Design review of the part built by this model. Coordinates are the model's own, in mm. Face numbers are marked on the shaded views. A direction names the side the tool comes from. Give positions to 0.01 mm unless a question says otherwise; leave off trailing zeros. Loops run counter-clockwise (first coordinate to the right, second up) from the corner with the lowest first, then second, coordinate; pieces in that order, holes last. Notation, with made-up numbers: M 72.5,77.25 L 127.5,77.25 A22 ccw 127.5,99.25 Z; hole C 18.5,14 d6. An arc over 180 degrees is marked long. Use one line per item in the form item = value. Start each with the question number.
from build123d import *

# Parameters (mm, degrees)
F0_W     = 22
F0_H     = 10
F1_DEPTH = 10
F2_R     = 1.65
F2_W     = 7
F2_H     = 4
F3_DEPTH = 10.001
F4_R     = 4.99999


# Not quite as in the source:
# - a fillet or chamfer is up to 0.001 mm smaller than in the source, because OpenCascade refuses the exact size


with BuildPart() as f1:
    # F0 (on Top) → F1 (new body)
    with BuildSketch(Plane.XY):
        Rectangle(F0_W, F0_H)
    extrude(amount=F1_DEPTH)

    # F2 (on face) → F3 (cut, through all)
    with BuildSketch(Plane.XY.offset(10)):
        with Locations((-7.5, 0)):
            Circle(F2_R)
        with Locations((7.5, 0)):
            Circle(F2_R)
        Rectangle(F2_W, F2_H)
    extrude(amount=-F3_DEPTH, mode=Mode.SUBTRACT)

    # F4 (radius 5 in the source; OpenCascade refuses exactly that, so slightly less here)
    f4_edges = [f1.edges().sort_by_distance(p)[0] for p in [
        (-11, 5, 5),
        (-11, -5, 5),
        (11, 5, 5),
        (11, -5, 5),
    ]]
    fillet(f4_edges, radius=F4_R)


solid = f1.part
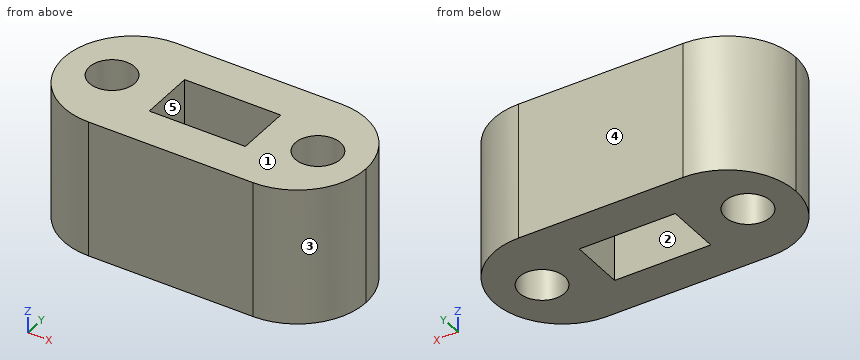
Q1. Take a section at A-A on x = 1. Give the boundary of the cut face in (y, z).
Q2. For the marked faces 4 and 5, list the 3-axis set-ups (+Z, -Z, +X, -X, +Y, -Y) from which the entire face can be reached by the end or side of a thin tool; tool diameter is ignored.
Q3. Take a section at C-C on y = 0.5. Give the boundary of the cut face in (x, z).
Q4. Wall thickness on probe 1 along X at (y, z) = (-1, 3.25); probe 2 along X at (y, z) = (1.5, 8); probe 3 along Y at (x, z) = (-0.5, 9): over which ranges is each line inside the solid? List them lowest first.
Q5. Take a section at B-B on z = 8.25. State how many separate pieces and enclosed holes the cut face has, plus the area to 3 significant figures.
Q6. The part is to be moulded in two halves that separate along X. For the marked faces 1, 2 and 3, say which applies: pulls with the +X half, pulls with the -X half, needs draft (parallel to the pull), parting line crosses it, or undercut.
Q7. Take a section at D-D on x = -6.75. Give the boundary of the cut face in (y, z).
Response values:
q1.outline = M -5,0 L -2,0 L -2,10 L -5,10 Z; M 2,0 L 5,0 L 5,10 L 2,10 Z
q2.face_4 = +Z, -Z, +X, -X, +Y
q2.face_5 = +Z, -Z
q3.outline = M -10.97,0 L -9.07,0 L -9.07,10 L -10.97,10 Z; M -5.93,0 L -3.5,0 L -3.5,10 L -5.93,10 Z; M 3.5,0 L 5.93,0 L 5.93,10 L 3.5,10 Z; M 9.07,0 L 10.97,0 L 10.97,10 L 9.07,10 Z
q4.probe_1 = -10.9 to -8.81, -6.19 to -3.5, 3.5 to 6.19, 8.81 to 10.9
q4.probe_2 = -10.77 to -8.19, -6.81 to -3.5, 3.5 to 6.81, 8.19 to 10.77
q4.probe_3 = -5 to -2, 2 to 5
q5.separate_pieces = 1
q5.enclosed_holes = 3
q5.area = 153 mm^2
q6.face_1 = needs draft
q6.face_2 = undercut
q6.face_3 = pulls with the +X half
q7.outline = M -4.94,0 L -1.47,0 L -1.47,10 L -4.94,10 Z; M 1.47,0 L 4.94,0 L 4.94,10 L 1.47,10 Z
